```python
from build123d import *

# Parameters (mm, degrees)
SKETCH1_W           = 25.4
SKETCH1_H           = 2.921
BOSS_EXTRUDE1_DEPTH = 2.921


with BuildPart() as part:
    # Sketch1 → Boss-Extrude1 (new body)
    with BuildSketch(Plane(origin=(0, 0, 0), x_dir=(1, 0, 0), z_dir=(0, 1, 0))):
        with BuildLine():
            Line((2.921, 0), (47.879, 0))
            Line((47.879, 0), (47.879, 12.7))
            Line((47.879, 12.7), (50.8, 12.7))
            Line((50.8, 12.7), (50.8, 21.640420504))
            ThreePointArc((50.8, 21.640420504), (47.21225, 22.225), (50.8, 22.809579496))
            Line((50.8, 22.809579496), (50.8, 31.75))
            Line((50.8, 31.75), (47.879, 31.75))
            Line((47.879, 31.75), (47.879, 44.45))
            Line((47.879, 44.45), (2.921, 44.45))
            Line((2.921, 44.45), (2.921, 31.75))
            Line((2.921, 31.75), (0, 31.75))
            Line((0, 31.75), (0, 22.809579496))
            ThreePointArc((0, 22.809579496), (3.58775, 22.225), (0, 21.640420504))
            Line((0, 21.640420504), (0, 12.7))
            Line((0, 12.7), (2.921, 12.7))
            Line((2.921, 12.7), (2.921, 0))
        make_face()
        with Locations((25.4, 4.6355)):
            Rectangle(SKETCH1_W, SKETCH1_H, mode=Mode.SUBTRACT)
    extrude(amount=BOSS_EXTRUDE1_DEPTH)


solid = part.part
```
Here's how the part is built. I have some questions about the finished solid (model axes, mm). A direction names the side the tool comes from. Coordinates: 2 decimals unless noted, no trailing zeros. Order: outer loops, then holes, each group sorted by start corner. A loop starts at its lowest first (then second) coordinate and runs counter-clockwise, first axis right, second up. Notation, with made-up numbers: (61.25, 75) - (79.25, 75) arc R19 ccw to (79.25, 100) - close; hole circle Ø1 at (-14.75, 50.25). An arc over 180 degrees is marked (long way). One line per question, with ' | ' between items.
(1) Will these pins go through, and if not, where does the flat tip stop? pin 1 (1.5 mm diameter, centred on y = 1.5, z = -7.5, fed in from +X); pin 2 (1.5 mm diameter, centred on y = 1.5, z = -4.5, fed in from -X); pin 3 (1.5 mm diameter, centred on x = 1.5, y = 2, fed in from +Z).
Report:
pin 1: stops at x = 47.88 | pin 2: stops at x = 2.92 | pin 3: stops at z = -12.7
(2) Suppose I cut it at A-A on x = 21.5. List the corners of the cut face in (y, z) for me (3 decimals), and give its area (3 significant figures).
Report:
outline: (0, -44.45) - (2.921, -44.45) - (2.921, -6.096) - (0, -6.096) - close; (0, -3.175) - (2.921, -3.175) - (2.921, 0) - (0, 0) - close | area: 121 mm2
(3) If we mould it in two halves opening along X, with no side actions, what happens to faces 4 (the flat face through (47.879, 1, -6)), 5 (the flat face through (25, 1, -3.175)), 6 (the flat face through (2.921, 1, -6)), 7 (the flat face through (25, 0, -23))? For each: pulls with the +X half, pulls with the -X half, needs draft (parallel to the pull), parting line crosses it, or undercut.
Report:
face 4: pulls with the +X half | face 5: undercut | face 6: pulls with the -X half | face 7: needs draft
(4) If I drill on L1, parallel to Z at x = 15, y = 1.4 (3 decimals); L2, parallel to X at y = 1.55, z = -6; L3, parallel to X at y = 2, z = -38, over which ranges is the centre line in solid material (lowest first)?
Report:
L1: z = -44.45 to -6.096, -3.175 to 0 | L2: x = 2.92 to 12.7, 38.1 to 47.88 | L3: x = 2.92 to 47.88
(5) For faces 1 (the flat face through (38.1, 1, -5)), 2 (the flat face through (2.921, 1, -38)), 3 (the flat face through (49, 1, -12.7)), which set-ups out of +Z, -Z, +X, -X, +Y, -Y let a thin tool reach every point of the face, with its end or its side?
Report:
face 1: +Y, -Y | face 2: -Z, -X, +Y, -Y | face 3: +Z, +X, +Y, -Y
(6) Suppose I cut it at C-C on z = -12. List the corners of the cut face in (x, y) for me, and give its area (3 significant figures).
Report:
outline: (2.92, 0) - (47.88, 0) - (47.88, 2.92) - (2.92, 2.92) - close | area: 131 mm2
